Here's how the part is built. I have some questions about the finished solid (model axes, mm). Face numbers are marked on the shaded views. A direction names the side the tool comes from. Round coordinates to 2 decimals unless told otherwise and drop trailing zeros. Order: outer loops, then holes, each group sorted by start corner. A loop starts at its lowest first (then second) coordinate and runs counter-clockwise, first axis right, second up. Notation, with made-up numbers: (-25.75, 53.25) - (-6.75, 53.25) arc R15 cw to (-6.75, 71.25) - close; hole circle Ø6 at (64.25, -37.75). An arc over 180 degrees is marked (long way). One line per item, written item: value.
from build123d import *

# Parameters (mm, degrees)
F0_W     = 185
F0_H     = 250
F0_W_2   = 181
F0_H_2   = 246
F1_DEPTH = 50
F2_DEPTH = 2
F3_R     = 5
F4_R     = 5
F5_R     = 15
F6_DEPTH = 25
F7_R     = 0.99999


# Not quite as in the source:
# - a fillet or chamfer is up to 0.001 mm smaller than in the source, because OpenCascade refuses the exact size


with BuildPart() as f1:
    # F0 (on Top) → F1 (new body)
    with BuildSketch(Plane.XY):
        Rectangle(F0_W, F0_H)
        Rectangle(F0_W_2, F0_H_2, mode=Mode.SUBTRACT)
    extrude(amount=F1_DEPTH)

    # F0 (on Top) → F2 (join)
    with BuildSketch(Plane.XY):
        Rectangle(F0_W, F0_H)
        Rectangle(F0_W_2, F0_H_2, mode=Mode.SUBTRACT)
        Rectangle(F0_W_2, F0_H_2)
    extrude(amount=F2_DEPTH)

    # F3
    f3_edges = [f1.edges().sort_by_distance(p)[0] for p in [
        (92.5, 125, 25),
        (-92.5, 125, 25),
        (90.5, 123, 26),
        (-90.5, 123, 26),
        (-90.5, -123, 26),
        (-92.5, -125, 25),
        (92.5, -125, 25),
        (90.5, -123, 26),
    ]]
    fillet(f3_edges, radius=F3_R)

    # F4
    f4_edges = [f1.edges().sort_by_distance(p)[0] for p in [
        (-90.5, 0, 2),
        (-89.035534, -121.535534, 2),
        (-89.035534, 121.535534, 2),
        (0, -123, 2),
        (0, 123, 2),
        (89.035534, -121.535534, 2),
        (89.035534, 121.535534, 2),
        (90.5, 0, 2),
    ]]
    fillet(f4_edges, radius=F4_R)

    # F5 (on face) → F6 (cut)
    with BuildSketch(Plane.XZ.offset(125)):
        with Locations((0, 50)):
            Circle(F5_R)
    extrude(amount=-F6_DEPTH, mode=Mode.SUBTRACT)

    # F7 (radius 1 in the source; OpenCascade refuses exactly that, so slightly less here)
    f7_edges = [f1.edges().sort_by_distance(p)[0] for p in [
        (0, -123, 35),
        (0, -125, 35),
    ]]
    fillet(f7_edges, radius=F7_R)


solid = f1.part
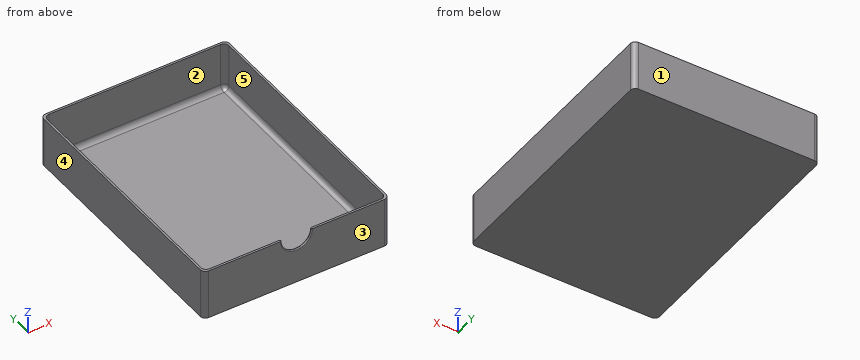
Q1. Will this pin go through, and if not, where does the flat tip stop? pin 1 (10 mm diameter, centred on x = 15, y = 19.5, fed in from +Z).
Results list:
pin 1: z = 2
Q2. If I drill on line 1 along Y through (x, z) = (85.5, 38.5); line 2 along X through (y, z) = (-101.5, 25); line 3 along Z through (x, y) = (-63.5, -69), over which ranges is the centre line in solid material (lowest first)?
Results list:
line 1: -125 to -123, 123 to 125
line 2: -92.5 to -90.5, 90.5 to 92.5
line 3: 0 to 2
Q3. Which directions (+Z, -Z, +X, -X, +Y, -Y) give clear straight access to the entire face, cutting with the end or side of a thin tool? Please do the marked faces 1 and 2.
Results list:
face 1: +Z, -Z, +X, -X, +Y
face 2: +Z
Q4. We'd pull the mould along X, two halves only. Please class the marked faces 3, 4 and 5: released by +X, released by -X, zero draft, split by the parting line, or undercut.
Results list:
face 3: zero draft
face 4: released by -X
face 5: undercut
Q5. If we section it at B-B, the plane x = 50.5: Please give me the cut outline in (y, z).
Results list:
outline: (-125, 0) - (125, 0) - (125, 50) - (123, 50) - (123, 7) arc R5 cw to (118, 2) - (-118, 2) arc R5 cw to (-123, 7) - (-123, 50) - (-125, 50) - close
Q6. If we section it at C-C, the plane y = 97: Please give me the cut outline in (x, z), then the cut area to 3 significant figures.
Results list:
outline: (-92.5, 0) - (92.5, 0) - (92.5, 50) - (90.5, 50) - (90.5, 7) arc R5 cw to (85.5, 2) - (-85.5, 2) arc R5 cw to (-90.5, 7) - (-90.5, 50) - (-92.5, 50) - close
area: 573 mm²
Q7. If we section it at A-A, the plane z = 22.5: Please give me the cut outline in (x, y).
Results list:
outline: (-92.5, -120) arc R5 ccw to (-87.5, -125) - (87.5, -125) arc R5 ccw to (92.5, -120) - (92.5, 120) arc R5 ccw to (87.5, 125) - (-87.5, 125) arc R5 ccw to (-92.5, 120) - close; hole (-90.5, -118) arc R5 ccw to (-85.5, -123) - (85.5, -123) arc R5 ccw to (90.5, -118) - (90.5, 118) arc R5 ccw to (85.5, 123) - (-85.5, 123) arc R5 ccw to (-90.5, 118) - close
